Autodesk Fusion 360 part; units mm, degrees
sketch "Sketch1" plane through (0, 0, 0) normal (0, 0, 1) x (1, 0, 0)
  line L0 (0, 0) -> (26.3, 0)
  line L1 (26.3, 0) -> (26.3, 30)
  line L2 (26.3, 30) -> (0, 30)
  line L3 (0, 30) -> (0, 0)
  line L4 (2, 28) -> (24.3, 28)
  line L5 (24.3, 28) -> (24.3, 2)
  line L6 (24.3, 2) -> (2, 2)
  line L7 (2, 2) -> (2, 28)
  line L8 (4, 26) -> (22.3, 26)
  line L9 (22.3, 26) -> (22.3, 4)
  line L10 (22.3, 4) -> (4, 4)
  line L11 (4, 4) -> (4, 26)
  dimension "d1" = 26.3
  dimension "d2" = 30
  dimension "d3" = 2
  dimension "d4" = 2
  dimension "d5" = 2
  dimension "d6" = 2
  dimension "d7" = 2
  dimension "d8" = 2
  dimension "d9" = 2
  dimension "d10" = 2
  dimension "d45" = 17.3
extrude "Extrude2" add sketch "Sketch1" along normal blind 1.5 makes body 1 at (10.1, 18.6667, 0) makes body 2 at (25.6333, 10.6667, 0)
extrude "Extrude1" add sketch "Sketch1" along normal blind 3.12 contours L4 L5 L6 L7 bodies 1 2
sketch "Sketch2" plane through (0, 0, 1.5) normal (0, 0, 1) x (-1, 0, 0)
  line L0 (-6.9, -22.5) -> (-9.4, -22.5)
  line L1 (-9.4, -22.5) -> (-9.4, -7)
  line L2 (-9.4, -7) -> (-6.9, -7)
  line L3 (-6.9, -7) -> (-6.9, -22.5)
  line L4 (-4, -4) -> (-22.3, -4)
  line L5 (-22.3, -4) -> (-22.3, -26)
  line L6 (-22.3, -26) -> (-4, -26)
  line L7 (-4, -26) -> (-4, -4)
  line L8 (-24.3, -2) -> (-2, -2)
  line L9 (-2, -2) -> (-2, -28)
  line L10 (-2, -28) -> (-24.3, -28)
  line L11 (-24.3, -28) -> (-24.3, -2)
  line L12 (0, -30) -> (0, 0)
  line L13 (0, 0) -> (-26.3, 0)
  line L14 (-26.3, 0) -> (-26.3, -30)
  line L15 (-26.3, -30) -> (0, -30)
  line L16 (-4.4, -23) -> (-4.4, -7)
  dimension "d15" = 15.5
  dimension "d16" = 2.5
  dimension "d39" = 2.9
  dimension "d40" = 6.9
  dimension "d41" = 4.9
  dimension "d43" = 4.4
  dimension "d44" = 2.5
extrude "Extrude3" cut sketch "Sketch2" against normal blind 3 contours L0 L1 L2 L3 bodies 1
sketch "Sketch3" plane through (0, 0, 0) normal (0, -1, 0) x (1, 0, 0)
  line L0 (0, 0) -> (26.3, 0)
  line L1 (26.3, 0) -> (26.3, 1.5)
  line L2 (26.3, 1.5) -> (0, 1.5)
  line L3 (0, 1.5) -> (0, 0)
  line L4 (0, 1.5) -> (-9.9853, -8.4853)
  line L5 (-9.9853, -8.4853) -> (-7.864, -10.6066)
  line L6 (-7.864, -10.6066) -> (2.7426, 0)
  dimension "d21" = 3
  dimension "d32" = 15
  dimension "d35" = 135
extrude "Extrude4" add sketch "Sketch3" against normal blind 30 contours L0 L3 L4 L5 L6 bodies 1
sketch "Sketch4" plane through (-0.75, 0, 0.75) normal (-0.7071, 0, 0.7071) x (0, -1, 0)
  line L0 (0, -13.0607) -> (0, 1.0607)
  line L1 (0, 1.0607) -> (-30, 1.0607)
  line L2 (-30, 1.0607) -> (-30, -13.0607)
  line L3 (-30, -13.0607) -> (0, -13.0607)
  circle A0 centre (-20, -7.9903) radius 1.6
  circle A1 centre (-10, -7.9903) radius 1.6
  dimension "d24" = 3.2
  dimension "d25" = 3.2
  dimension "d26" = 10
  dimension "d27" = 10
  dimension "d29" = 9.051
extrude "Extrude5" cut sketch "Sketch4" against normal blind 5 contours A0 | A1 bodies 1
fillet "Fillet2" radius 6 1 edges at (2.7426, 15, 0) on bodies 1
component "Component" placed x (1, 0, 0) y (0, 1, 0) z (0, 0, 1) at (0, 0, 0)
equation "d4 = d3"
equation "d5 = d3"
equation "d6 = d3"
equation "d8 = d7"
equation "d9 = d7"
equation "d10 = d7"
equation "d11 = 1.5 mm + 1.62 mm"
equation "d25 = d24"
equation "d27 = ( 30 mm - d26 ) / 2"
equation "d29 = Linear Dimension-4"
equation "d35 = Angular Dimension-2"
Work out the finished part from the listing and answer in its coordinate system (mm). A direction names the side the tool comes from. Give positions to 0.01 mm unless a question says otherwise; leave off trailing zeros. Loops run counter-clockwise (first coordinate to the right, second up) from the corner with the lowest first, then second, coordinate; pieces in that order, holes last. Notation, with made-up numbers: (49.5, 34) -> (72.5, 34) arc R9 ccw to (72.5, 41) -> close; hole circle Ø3 at (-1.5, 19.25). An arc over 180 degrees is marked (long way). Put each result on its own line as item: value. Start each with the question number.
Item 1: Find the intervals of material crossed by L1, parallel to Y at x = 7.5, z = 1.75; L2, parallel to Z at x = 14, y = 13.5; L3, parallel to Z at x = 23.5, y = 16.25, in increasing order. Write a range as [from, to].
Item 2: The part is cut by section D-D (y = 13.5). Give the vertices of the cut face in (x, z), then the cut area to 3 significant figures.
Item 3: The part is cut by section C-C (y = 20). Give the vertices of the cut face in (x, z).
Item 4: The part is cut by section A-A (x = 6). Give the vertices of the cut face in (y, z), then the cut area to 3 significant figures.
Item 5: The mould has two halves that part along Y. Classify faces 4 (the face through (8, 22.5, 1)), 5 (the face through (13, 28, 2)), 6 (the face through (16, 15, 0)): released by +Y, released by -Y, zero draft, split by the parting line, or undercut.
Item 6: Each of these flat-tipped pins is pushed along its axis until it touches: P1, Ø0.8, axis at y = 19.5, z = 2, coming from the -X side; P2, Ø1.5, axis at y = 18, z = -3.5, coming from the +X side; P3, Ø1.5, axis at x = -4.5, y = 4.5, coming from the +Z side. Where does it stop, or does it pass through?
Item 7: Which of the six approach directions +Z, -Z, +X, -X, +Y, -Y give full straight-line access (tool end or side, diameter ignored) to faces 1 (the face through (13, 4, 2)), 2 (the face through (6.9, 15, 1)), 3 (the face through (24.3, 15, 2))?
Item 8: The part is cut by section B-B (z = 0.5). Give the vertices of the cut face in (x, y), then the cut area to 3 significant figures.
Answers below:
1. L1: [2, 4], [26, 28]
1. L2: [0, 1.5]
1. L3: [0, 3.12]
2. outline: (-9.99, -8.49) -> (-7.86, -10.61) -> (0.99, -1.76) arc R6 cw to (5.23, 0) -> (6.9, 0) -> (6.9, 1.5) -> (4, 1.5) -> (4, 3.12) -> (2, 3.12) -> (2, 1.5) -> (0, 1.5) -> close; (9.4, 0) -> (26.3, 0) -> (26.3, 1.5) -> (24.3, 1.5) -> (24.3, 3.12) -> (22.3, 3.12) -> (22.3, 1.5) -> (9.4, 1.5) -> close
2. area: 84.6 mm2
3. outline: (-9.99, -8.49) -> (-7.86, -10.61) -> (-5.41, -8.15) -> (-7.53, -6.03) -> close; (-5.27, -3.77) -> (-3.15, -5.89) -> (0.99, -1.76) arc R6 cw to (5.23, 0) -> (6.9, 0) -> (6.9, 1.5) -> (4, 1.5) -> (4, 3.12) -> (2, 3.12) -> (2, 1.5) -> (0, 1.5) -> close; (9.4, 0) -> (26.3, 0) -> (26.3, 1.5) -> (24.3, 1.5) -> (24.3, 3.12) -> (22.3, 3.12) -> (22.3, 1.5) -> (9.4, 1.5) -> close
4. outline: (0, 0) -> (30, 0) -> (30, 1.5) -> (28, 1.5) -> (28, 3.12) -> (26, 3.12) -> (26, 1.5) -> (4, 1.5) -> (4, 3.12) -> (2, 3.12) -> (2, 1.5) -> (0, 1.5) -> close
4. area: 51.5 mm2
5. face 4: undercut
5. face 5: released by +Y
5. face 6: zero draft
6. P1: x = 2
6. P2: x = -0.01
6. P3: z = -2.25
7. face 1: +Z
7. face 2: +Z, -Z
7. face 3: +Z, +X, +Y, -Y
8. outline: (-1, 0) -> (26.3, 0) -> (26.3, 30) -> (-1, 30) -> close; hole (6.9, 7) -> (9.4, 7) -> (9.4, 22.5) -> (6.9, 22.5) -> close
8. area: 780 mm2
